```python
from build123d import *

# Parameters (mm, degrees)
SKETCH1_W                = 28.5
SKETCH1_H                = 23
CENTRE_BLOCK_DEPTH       = 128
TOP_CYLINDER_DEPTH       = 7
TOP_CYLINDER_DEPTH_BACK  = 90
CUT_REVOLVE2_ANGLE       = 180
NOSE_DEPTH               = 131.828370394
T_CROSS_REACH            = 134.885
SKETCH6_R                = 12
BARREL_DEPTH             = 7
SIDE_CYLINDER_DEPTH      = 128
CUT_REVOLVE1_ANGLE       = 180
SKETCH8_R                = 2.75
BACK_HOLE_DEPTH          = 5
SKETCH15_R               = 2.75
CUT_EXTRUDE6_DEPTH       = 10
FILLET2_R                = 1
SKETCH16_R               = 6.5
CUT_EXTRUDE7_DEPTH       = 20
SKETCH21_W               = 152.585030794
SKETCH21_H               = 42.838852891
CUT_EXTRUDE10_DEPTH      = 133.885289011
SKETCH23_R               = 2.75
CUT_EXTRUDE11_DEPTH      = 5
SKETCH24_R               = 2.75
BOTTOM_MOUNT_HOLES_DEPTH = 5


with BuildPart() as part:
    # Sketch1 → Centre block (new body)
    with BuildSketch(Plane.XY):
        Rectangle(SKETCH1_W, SKETCH1_H)
    extrude(amount=CENTRE_BLOCK_DEPTH)

    # Sketch3 → top cylinder (add, two sides: drawn at the far end of the back side and taken through both)
    with BuildSketch(Plane(origin=(0, 0, 0), x_dir=(-1, 0, 0), z_dir=(0, 0, -1)).offset(-TOP_CYLINDER_DEPTH_BACK)):
        with BuildLine():
            Line((-10, 11.5), (10, 11.5))
            ThreePointArc((10, 11.5), (0, 21.5), (-10, 11.5))
        make_face()
    extrude(amount=TOP_CYLINDER_DEPTH + TOP_CYLINDER_DEPTH_BACK)

    # Sketch9 → Cut-Revolve2 (revolve, cut)
    with BuildSketch(Plane(origin=(0, 11.5, 0), x_dir=(1, 0, 0), z_dir=(0, 1, 0))):
        Polygon((10, -78), (10, -81.888582416), (23.187071127, -81.888582416), (23.187071127, -74.052631606), (23.187071127, 0), (10, 0), (10, -8), (9.5, -8), (9.5, -8.5), (10, -8.5), (10, -11.5), (8, -13.5), (8, -16.5), (10, -18.5), (10, -21.5), (9.5, -21.5), (9.5, -22), (10, -22), (10, -25), (9.5, -25), (9.5, -25.5), (10, -25.5), (10, -28.5), (8, -30.5), (8, -33.5), (10, -35.5), (10, -38.5), (8, -38.5), (8, -41.5), (10, -43.5), (10, -48.5), (8, -48.5), (8, -51.5), (10, -53.5), (10, -58.5), (8, -58.5), (8, -60.3), (8, -61.5), (10, -63.5), (10, -68.5), (8, -68.5), (8, -70.3), (8, -71.5), (10, -73.5), (10, -74.052631606), (10, -77.5), (9.5, -77.5), (9.5, -78), align=None)
    revolve(axis=Axis((0, 11.5, -7), (0, 0, 1)), revolution_arc=CUT_REVOLVE2_ANGLE, mode=Mode.SUBTRACT)

    # Sketch4 → nose (cut, through all)
    with BuildSketch(Plane.XZ.offset(-11.5)):
        with BuildLine():
            Line((-3.25, -7), (-3.25, -2))
            ThreePointArc((-3.25, -2), (-3.835786438, -0.585786438), (-5.25, 0))
            Line((-5.25, 0), (-10, 0))
            Line((-10, 0), (-10, -7))
            Line((-10, -7), (-3.25, -7))
        make_face()
        with BuildLine():
            Line((3.75, -7), (3.75, -2))
            ThreePointArc((3.75, -2), (4.335786438, -0.585786438), (5.75, 0))
            Line((5.75, 0), (10, 0))
            Line((10, 0), (10, -7))
            Line((10, -7), (3.75, -7))
        make_face()
    extrude(amount=-NOSE_DEPTH, mode=Mode.SUBTRACT)

    # t cross: up to this face of the body (flat: up to its plane)
    t_cross_end = Plane(part.part.faces().sort_by_distance((-14.25, 0, 64))[0])
    # Sketch5 → t cross (add, up to the picked face)
    with BuildSketch(Plane(origin=(14.25, 0, 0), x_dir=(0, 0, -1), z_dir=(1, 0, 0)), mode=Mode.PRIVATE) as t_cross_sk1:
        with BuildLine():
            Line((-101, 11.5), (-81, 11.5))
            ThreePointArc((-81, 11.5), (-91, 21.5), (-101, 11.5))
        make_face()
    t_cross_tool1 = split(extrude(t_cross_sk1.sketch, amount=-T_CROSS_REACH, mode=Mode.PRIVATE), bisect_by=t_cross_end, keep=Keep.BOTH, mode=Mode.PRIVATE)
    add(t_cross_tool1.solids().sort_by(Axis((14.25, 15.744132, 91), (-1, 0, 0)))[0])

    # Sketch6 → Barrel (add)
    with BuildSketch(Plane(origin=(0, 0, 0), x_dir=(-1, 0, 0), z_dir=(0, 0, -1))):
        with Locations((0, 0.5)):
            Circle(SKETCH6_R)
    extrude(amount=BARREL_DEPTH)

    # Sketch2 → side cylinder (add)
    with BuildSketch(Plane(origin=(0, 0, 0), x_dir=(-1, 0, 0), z_dir=(0, 0, -1))):
        with BuildLine():
            Line((14.25, 10), (14.25, -10))
            ThreePointArc((14.25, -10), (24.25, 0), (14.25, 10))
        make_face()
    extrude(amount=-SIDE_CYLINDER_DEPTH)

    # Sketch7 → Cut-Revolve1 (revolve, cut)
    with BuildSketch(Plane(origin=(-14.25, 0, 0), x_dir=(0, 0, -1), z_dir=(1, 0, 0))):
        Polygon((-51, -10), (-51, -9), (-51.5, -9), (-51.5, -10), (-55.5, -10), (-57.5, -8), (-58.77482941, -8), (-60.5, -8), (-60.5, -10), (-64.5, -10), (-66.5, -8), (-67.77482941, -8), (-69.5, -8), (-69.5, -10), (-73.5, -10), (-75.5, -8), (-76.77482941, -8), (-78.5, -8), (-78.5, -10), (-82.5, -10), (-84.5, -8), (-85.77482941, -8), (-87.5, -8), (-87.5, -10), (-91.5, -10), (-93.5, -8), (-94.77482941, -8), (-96.5, -8), (-96.5, -10), (-100.5, -10), (-102.5, -8), (-105.5, -8), (-107.5, -10), (-110.5, -10), (-110.5, -9), (-111, -9), (-111, -10), (-114, -10), (-114, -9), (-114.5, -9), (-114.5, -10), (-117.5, -10), (-119.5, -8), (-122.65, -8), (-124.65, -10), (-124.65, -14.812383498), (-117.5, -14.812383498), (0, -14.812383498), (0, -10), align=None)
    revolve(axis=Axis((-14.25, 0, 135.382259058), (0, 0, -1)), revolution_arc=CUT_REVOLVE1_ANGLE, mode=Mode.SUBTRACT)

    # Sketch8 → Back hole (cut)
    with BuildSketch(Plane.XY.offset(128)):
        Circle(SKETCH8_R)
    extrude(amount=-BACK_HOLE_DEPTH, mode=Mode.SUBTRACT)

    # Sketch15 → Cut-Extrude6 (cut)
    with BuildSketch(Plane(origin=(14.25, 0, 0), x_dir=(0, 0, -1), z_dir=(1, 0, 0))):
        with Locations((-91, 11.5)):
            Circle(SKETCH15_R)
        with Locations((-91, -6.5)):
            Circle(SKETCH15_R)
    extrude(amount=-CUT_EXTRUDE6_DEPTH, mode=Mode.SUBTRACT)

    # Fillet2
    fillet2_edges = [part.edges().sort_by_distance(p)[0] for p in [
        (-14.25, 11.5, 40.5),
        (14.25, 11.5, 40.5),
        (14.25, -11.5, 64),
        (-14.25, -11.5, 64),
        (-14.25, 11.5, 114.5),
        (14.25, 11.5, 114.5),
    ]]
    fillet(fillet2_edges, radius=FILLET2_R)

    # Sketch16 → Cut-Extrude7 (cut)
    with BuildSketch(Plane(origin=(0, 0, -7), x_dir=(-1, 0, 0), z_dir=(0, 0, -1))):
        Circle(SKETCH16_R)
    extrude(amount=-CUT_EXTRUDE7_DEPTH, mode=Mode.SUBTRACT)

    # Sketch21 → Cut-Extrude10 (cut, through all)
    with BuildSketch(Plane.ZY.offset(14.25)):
        with Locations((64.09795532, 3.365381731)):
            Rectangle(SKETCH21_W, SKETCH21_H)
    extrude(amount=CUT_EXTRUDE10_DEPTH, mode=Mode.SUBTRACT)

    # Sketch23 → Cut-Extrude11 (cut)
    with BuildSketch(Plane.ZY.offset(14.25)):
        with Locations((10, 0)):
            Circle(SKETCH23_R)
        with Locations((118, 0)):
            Circle(SKETCH23_R)
        with Locations((64, 0)):
            Circle(SKETCH23_R)
    extrude(amount=-CUT_EXTRUDE11_DEPTH, mode=Mode.SUBTRACT)

    # Sketch24 → Bottom Mount Holes (cut)
    with BuildSketch(Plane.XZ.offset(11.5)):
        with Locations(Location((0, 20, 0), (0, 0, 270))):
            Circle(SKETCH24_R)
        with Locations(Location((0, 90, 0), (0, 0, 270))):
            Circle(SKETCH24_R)
    extrude(amount=-BOTTOM_MOUNT_HOLES_DEPTH, mode=Mode.SUBTRACT)


solid = part.part
```
Can you work these out from the model? Positions are in its coordinate system, mm. A direction names the side the tool comes from. Give positions to 0.01 mm unless a question says otherwise; leave off trailing zeros. Write each loop counter-clockwise with the first axis right and the second up, starting at its lowest first coordinate (ties: lowest second). Pieces come first, ordered by that corner, then holes. Notation, with made-up numbers: (-23, 7.5) - (-3, 7.5) arc R21 ccw to (-3, 32.5) - close; hole circle Ø3 at (44, 63.25). An arc over 180 degrees is marked (long way). Write item = value, one per line. Start each with the question number.
1. Imagine slicing it at C-C (y = 1.5). Please give me the cut outline in (x, z).
2. Imagine slicing it at B-B (z = 10). Please give me the cut outline in (x, y).
3. Please list where these lines run through material, in increasing order: line 1 (Y direction, x = -13.15, z = 10); line 2 (Z direction, x = -2.25, y = -8.5); line 3 (Y direction, x = 0, z = 3).
4. Thinking about a two-plate mould opening in Y: for faces 1 (the face through (0, 21.3, 8.5)), 2 (the face through (-9.25, 0, 118)), 3 (the face through (0, 20, 72)), which applies, released by +Y, released by -Y, zero draft, split by the parting line, or undercut?
5. Imagine slicing it at D-D (z = 32). Please give me the cut outline in (x, y).
6. Imagine slicing it at A-A (z = 118). Please give me the cut outline in (x, y), and give its area (3 significant figures).
7. On a 3-axis mill with a long thin cutter (end or side, diameter ignored), from which of +Z, -Z, +X, -X, +Y, -Y can I reach the whole of each face in a straight line? I mean faces 4 (the face through (0, 21.3, 77.5)), 5 (the face through (11, 11.5, 40)), 6 (the face through (0, -6.5, 90)), 7 (the face through (-0.2, 21.5, 2.3)). Say none if no direction works.
8. For pin 1 (11.5 mm diameter, centred on x = 0, y = 0, fed in from -Z); pin 2 (3 mm diameter, centred on y = 0, z = 9.5, fed in from -X); pin 3 (8 mm diameter, centred on x = 2.5, y = 17, fed in from +Z), each with a flat end and sliding along its axis, tell me the tip position at first contact or that it passes through.
Worked answers:
q1.outline = (-14.25, 0) - (-11.96, 0) - (-11.96, -7) - (-6.32, -7) - (-6.32, 13) - (6.32, 13) - (6.32, -7) - (11.96, -7) - (11.96, 0) - (14.25, 0) - (14.25, 128) - (2.3, 128) - (2.3, 123) - (-2.3, 123) - (-2.3, 128) - (-14.25, 128) - (-14.25, 120.3) - (-9.25, 120.3) - (-9.25, 115.7) - (-14.25, 115.7) - (-14.25, 66.3) - (-9.25, 66.3) - (-9.25, 61.7) - (-14.25, 61.7) - (-14.25, 12.3) - (-9.25, 12.3) - (-9.25, 7.7) - (-14.25, 7.7) - close
q2.outline = (-14.25, -10.5) arc R1 ccw to (-13.25, -11.5) - (13.25, -11.5) arc R1 ccw to (14.25, -10.5) - (14.25, 10.5) arc R1 ccw to (13.25, 11.5) - (10, 11.5) arc R10 ccw to (-10, 11.5) - (-13.25, 11.5) arc R1 ccw to (-14.25, 10.5) - (-14.25, 2.75) - (-9.25, 2.75) - (-9.25, -2.75) - (-14.25, -2.75) - close; hole circle Ø13 at (0, 0)
q3.line_1 = -11.5 to -2.75, 2.75 to 11.5
q3.line_2 = -7 to 18.42, 21.58 to 88.42, 91.58 to 128
q3.line_3 = -11.5 to -6.5, 6.5 to 21.5
q4.face_1 = zero draft
q4.face_2 = undercut
q4.face_3 = released by +Y
q5.outline = (-14.25, -10.5) arc R1 ccw to (-13.25, -11.5) - (13.25, -11.5) arc R1 ccw to (14.25, -10.5) - (14.25, 10.5) arc R1 ccw to (13.25, 11.5) - (8, 11.5) arc R8 ccw to (-8, 11.5) - (-13.25, 11.5) arc R1 ccw to (-14.25, 10.5) - close
q6.outline = (-14.25, -10.5) arc R1 ccw to (-13.25, -11.5) - (13.25, -11.5) arc R1 ccw to (14.25, -10.5) - (14.25, 10.5) arc R1 ccw to (13.25, 11.5) - (-13.25, 11.5) arc R1 ccw to (-14.25, 10.5) - (-14.25, 2.75) - (-9.25, 2.75) - (-9.25, -2.75) - (-14.25, -2.75) - close
q6.area = 627 mm2
q7.face_4 = +Y
q7.face_5 = +X, +Y
q7.face_6 = -Y
q7.face_7 = -Z, +Y
q8.pin_1 = 13
q8.pin_2 = -9.25
q8.pin_3 = 100.89
